Verification items for this drawing (mm, ordinates from the low corner). Give positions to 0.01 mm unless a question says otherwise; leave off trailing zeros. Order: outer loops, then holes, each group sorted by start corner. A loop starts at its lowest first (then second) coordinate and runs counter-clockwise, first axis right, second up. Notation, with made-up numbers: (83.25, 76.25) - (138.25, 76.25) arc R24 ccw to (138.25, 97.25) - close; hole circle Ø6 at (-21, 33). An arc over 180 degrees is marked (long way). Put each result on its own line as item: value. Start each with the question number.
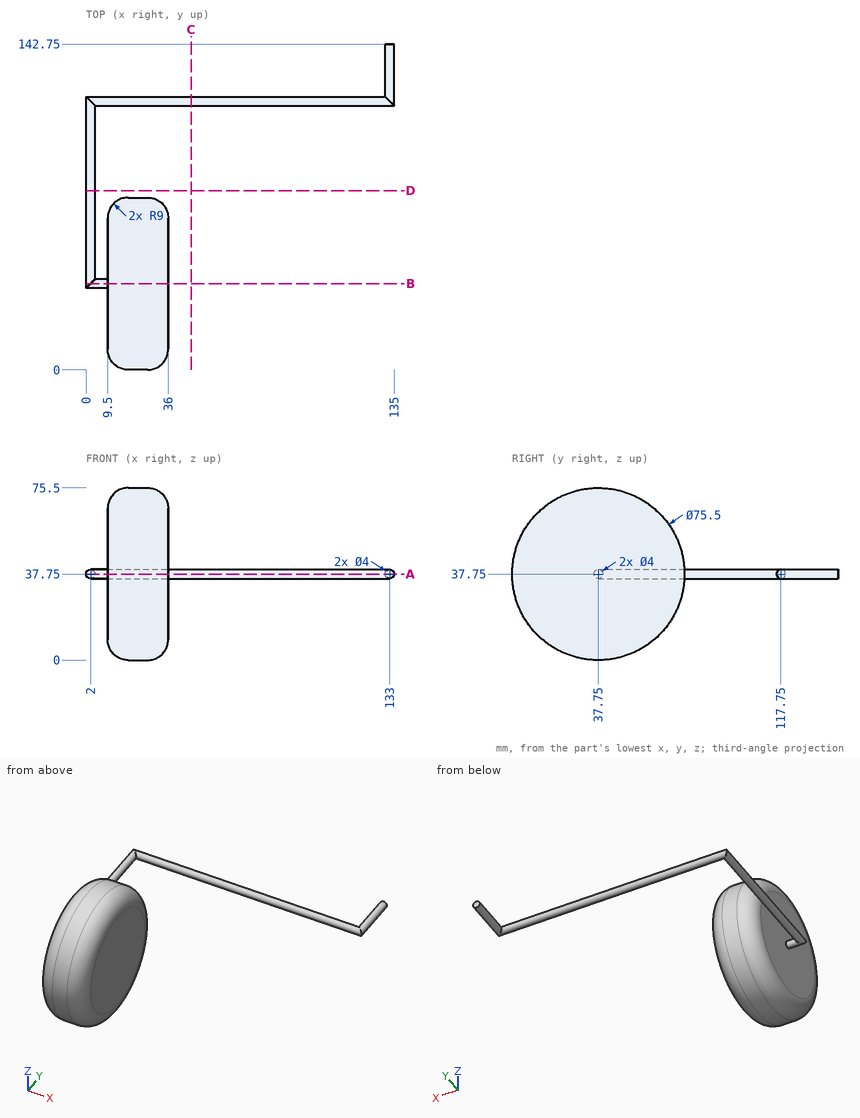
Item 1: Cross-section at C-C (x = 46). Enter the section's corners in (y, z), and give its area (3 significant figures).
Item 2: Cross-section at D-D (y = 78.5). Enter the section's corners in (x, z), and give its area (3 significant figures).
Item 3: Gauge pin test, flat ends, axial feed: pin 1 Ø8 at (x, y) = (62.5, 123.5) entering from -Z; pin 2 Ø1.5 at (y, z) = (49.5, 47.5) entering from +X. Record the tip position at first contact, or that the pin passes through.
Item 4: Cross-section at B-B (y = 37.75). Enter the section's corners in (x, z).
Item 5: Cross-section at A-A (z = 37.75). Enter the section's corners in (x, y), and give its area (3 significant figures).
Item 6: Thickness scan on line 1 along X through (y, z) = (31, 27.5); line 2 along X through (y, z) = (115.5, 39); line 3 along Y through (x, z) = (23.5, 11.5). Record the ranges inside material, lowest first.
Recorded:
1. outline: circle Ø4 at (117.75, 37.75)
1. area: 12.6 mm^2
2. outline: circle Ø4 at (2, 37.75)
2. area: 12.6 mm^2
3. pin 1: stops at z = 36.78
3. pin 2: stops at x = 36
4. outline: (2, 35.75) - (9.5, 35.75) - (9.5, 9) arc R9 ccw to (18.5, 0) - (27, 0) arc R9 ccw to (36, 9) - (36, 66.5) arc R9 ccw to (27, 75.5) - (18.5, 75.5) arc R9 ccw to (9.5, 66.5) - (9.5, 39.75) - (2, 39.75) arc R2 ccw to start
5. outline: (0, 35.75) - (9.5, 35.75) - (9.5, 9) arc R9 ccw to (18.5, 0) - (27, 0) arc R9 ccw to (36, 9) - (36, 66.5) arc R9 ccw to (27, 75.5) - (18.5, 75.5) arc R9 ccw to (9.5, 66.5) - (9.5, 39.75) - (4, 39.75) - (4, 115.75) - (135, 115.75) - (135, 142.75) - (131, 142.75) - (131, 119.75) - (0, 119.75) - close
5. area: 2,910 mm^2
6. line 1: x = 9.5 to 36
6. line 2: x = 0.44 to 3.56
6. line 3: y = 10.62 to 64.88
